```python
from build123d import *

# Parameters (mm, degrees)
BOSS_EXTRUDE1_DEPTH                        = 3
SKETCH4_R                                  = 2.250000000000006
CUT_EXTRUDE2_DEPTH                         = 3
MIRROR1_AT_THE_SECOND_PLANE_COPY_1_SKETC_R = 2.250000000000006
MIRROR1_AT_THE_SECOND_PLANE_COPY_1_DEPTH   = 3
FILLET4_R                                  = 1
CUT_EXTRUDE3_DEPTH                         = 1
SKETCH6_W                                  = 27.499999999999993
SKETCH6_H                                  = 27.999999999999996
CUT_EXTRUDE4_DEPTH                         = 1
CUT_EXTRUDE5_DEPTH                         = 3
SKETCH8_W                                  = 13.499999999999996
SKETCH8_H                                  = 13.700000000000003
CUT_EXTRUDE6_DEPTH                         = 1
SKETCH9_W                                  = 13.5
SKETCH9_H                                  = 3.5000000000000036
CUT_EXTRUDE7_DEPTH                         = 3
SKETCH10_W                                 = 13.499999999999996
SKETCH10_H                                 = 3.5000000000000036
SKETCH10_H_2                               = 3.5000000000000018
CUT_EXTRUDE8_DEPTH                         = 3
BOSS_EXTRUDE2_DEPTH                        = 23.5
CUT_EXTRUDE9_DEPTH                         = 29
SKETCH13_W                                 = 20.500000000000004
SKETCH13_H                                 = 6.0000000000000036
CUT_EXTRUDE10_DEPTH                        = 3
FILLET5_R                                  = 1
FILLET6_R                                  = 1
SKETCH14_W                                 = 20.8
SKETCH14_H                                 = 3.0000000000000036
CUT_EXTRUDE11_DEPTH                        = 1


with BuildPart() as part:
    # Sketch1 → Boss-Extrude1 (new body)
    with BuildSketch(Plane(origin=(0, 0, 0), x_dir=(1, 0, 0), z_dir=(0, 1, 0))):
        Polygon((-35, 35.00000000000001), (35, 35.00000000000001), (35.000000000000014, -34.99999999999999), (-35, -34.99999999999999), align=None)
    extrude(amount=BOSS_EXTRUDE1_DEPTH)

    # Sketch4 → Cut-Extrude2 (cut)
    with BuildSketch(Plane(origin=(0, 0, 0), x_dir=(-1, 0, 0), z_dir=(0, -1, 0))):
        with Locations(Location((30.500000000000004, -30.499999999999993, 0), (0, 0, 90))):
            Circle(SKETCH4_R)
    cut_extrude2 = extrude(amount=-CUT_EXTRUDE2_DEPTH, mode=Mode.SUBTRACT)

    # Mirror1: Cut-Extrude2 across plane
    add(cut_extrude2.mirror(Plane(origin=(0, 0, 0), x_dir=(0, 0, 1), z_dir=(1, 0, 0))), mode=Mode.SUBTRACT)

    # Mirror1 at the second plane: Cut-Extrude2 across plane
    add(cut_extrude2.mirror(Plane.XY), mode=Mode.SUBTRACT)

    # Mirror1 at the second plane copy 1 sketc → Mirror1 at the second plane copy 1 (cut)
    with BuildSketch(Plane.XZ):
        with Locations(Location((30.500000000000004, -30.499999999999993, 0), (0, 0, 90))):
            Circle(MIRROR1_AT_THE_SECOND_PLANE_COPY_1_SKETC_R)
    extrude(amount=-MIRROR1_AT_THE_SECOND_PLANE_COPY_1_DEPTH, mode=Mode.SUBTRACT)

    # Fillet4
    fillet4_edges = [part.edges().sort_by_distance(p)[0] for p in [
        (7.11e-15, 0, 34.99999999999999),
        (-35, 0, -7.11e-15),
        (0, 0, -35.00000000000001),
        (35.00000000000001, 0, -7.11e-15),
    ]]
    fillet(fillet4_edges, radius=FILLET4_R)

    # Sketch5 → Cut-Extrude3 (cut)
    with BuildSketch(Plane(origin=(0, 0, 0), x_dir=(-1, 0, 0), z_dir=(0, -1, 0))):
        Polygon((28.79465847473562, -24.725896818258043), (7.994658474735617, -24.725896818258047), (7.994658474735617, 20.774103181741953), (28.79465847473562, 20.774103181741957), align=None)
    extrude(amount=-CUT_EXTRUDE3_DEPTH, mode=Mode.SUBTRACT)

    # Sketch6 → Cut-Extrude4 (cut)
    with BuildSketch(Plane.XZ):
        with Locations((15.477858409688114, -6.209961428811168)):
            Rectangle(SKETCH6_W, SKETCH6_H)
    extrude(amount=-CUT_EXTRUDE4_DEPTH, mode=Mode.SUBTRACT)

    # Sketch7 → Cut-Extrude5 (cut)
    with BuildSketch(Plane(origin=(0, 1, 0), x_dir=(-1, 0, 0), z_dir=(0, -1, 0))):
        Polygon((-7.977858409688114, 15.209961428811162), (-22.977858409688114, 15.20996142881116), (-22.977858409688114, 20.209961428811166), (-7.977858409688114, 20.209961428811166), align=None)
    extrude(amount=-CUT_EXTRUDE5_DEPTH, mode=Mode.SUBTRACT)

    # Sketch8 → Cut-Extrude6 (cut)
    with BuildSketch(Plane.XZ):
        Polygon((-0.32931613637633694, 25.216207013959828), (13.170683863623664, 25.216207013959828), (13.170683863623664, 11.516207013959828), (-0.3293161363763353, 11.516207013959828), align=None)
        with Locations((23.356942305835496, 18.36620701395983)):
            Rectangle(SKETCH8_W, SKETCH8_H)
    extrude(amount=-CUT_EXTRUDE6_DEPTH, mode=Mode.SUBTRACT)

    # Sketch9 → Cut-Extrude7 (cut)
    with BuildSketch(Plane(origin=(0, 1, 0), x_dir=(-1, 0, 0), z_dir=(0, -1, 0))):
        with Locations((-6.420683863623664, -23.46620701395983)):
            Rectangle(SKETCH9_W, SKETCH9_H)
        Polygon((0.3293161363763353, -11.516207013959828), (-13.170683863623664, -11.51620701395983), (-13.170683863623664, -15.01620701395983), (0.3293161363763357, -15.016207013959828), align=None)
    extrude(amount=-CUT_EXTRUDE7_DEPTH, mode=Mode.SUBTRACT)

    # Sketch10 → Cut-Extrude8 (cut)
    with BuildSketch(Plane.XZ.offset(-1)):
        with Locations((23.356942305835496, 23.46620701395983)):
            Rectangle(SKETCH10_W, SKETCH10_H)
        with Locations((23.356942305835496, 13.266207013959828)):
            Rectangle(SKETCH10_W, SKETCH10_H_2)
    extrude(amount=-CUT_EXTRUDE8_DEPTH, mode=Mode.SUBTRACT)

    # Sketch11 → Boss-Extrude2 (add)
    with BuildSketch(Plane(origin=(0, 1, 0), x_dir=(-1, 0, 0), z_dir=(0, -1, 0))):
        Polygon((31.644658474735618, -26.345290910107266), (5.144658474735617, -26.34529091010727), (5.144658474735617, 5.654709089892729), (31.644658474735618, 5.654709089892732), align=None)
    extrude(amount=BOSS_EXTRUDE2_DEPTH)

    # Sketch12 → Cut-Extrude9 (cut)
    with BuildSketch(Plane(origin=(5.6e-16, 0, -5.654709089892728), x_dir=(-1, 0, -1e-16), z_dir=(1e-16, 0, -1))):
        Polygon((8.144658474735618, 1), (28.644658474735618, 1), (28.64465847473562, -19.5), (8.14465847473562, -19.5), align=None)
    extrude(amount=-CUT_EXTRUDE9_DEPTH, mode=Mode.SUBTRACT)

    # Sketch13 → Cut-Extrude10 (cut)
    with BuildSketch(Plane.XZ.offset(-1)):
        with Locations((-18.39465847473562, 20.345290910107273)):
            Rectangle(SKETCH13_W, SKETCH13_H)
    extrude(amount=-CUT_EXTRUDE10_DEPTH, mode=Mode.SUBTRACT)

    # Fillet5
    fillet5_edges = [part.edges().sort_by_distance(p)[0] for p in [
        (-5.144658474735617, -11.25, 26.34529091010727),
        (-31.644658474735618, -11.25, 26.345290910107266),
        (-5.144658474735617, -11.25, -5.654709089892729),
        (-31.644658474735618, -11.25, -5.654709089892732),
        (-28.64465847473562, -9.25, -5.654709089892731),
        (-18.39465847473562, -19.5, -5.65470908989273),
        (-8.144658474735618, -9.25, -5.654709089892729),
        (-18.394658474735618, -22.5, 26.345290910107266),
        (-5.144658474735617, -22.5, 10.34529091010727),
        (-18.394658474735618, -22.5, -5.65470908989273),
        (-31.644658474735618, -22.5, 10.345290910107268),
    ]]
    fillet(fillet5_edges, radius=FILLET5_R)

    # Fillet6
    fillet6_edges = [part.edges().sort_by_distance(p)[0] for p in [
        (-18.394658474735618, 0, 26.345290910107266),
        (-5.144658474735617, 0, 10.34529091010727),
        (-31.644658474735618, 0, 10.345290910107266),
        (-6.644658474735618, 0, -5.654709089892728),
        (-30.144658474735618, 0, -5.654709089892731),
        (-5.43755169354907, 0, 26.052397691293816),
        (-31.351765255922164, 0, 26.052397691293812),
        (-5.437551693549068, 0, -5.361815871079277),
        (-31.351765255922164, 0, -5.361815871079279),
        (-29.15823411660915, -8e-17, -5.528431782639838),
        (-7.631082832861968, 4e-17, -5.528431782639901),
    ]]
    fillet(fillet6_edges, radius=FILLET6_R)

    # Sketch14 → Cut-Extrude11 (cut)
    with BuildSketch(Plane.XZ):
        with Locations((-18.394658474735618, -22.274103181741957)):
            Rectangle(SKETCH14_W, SKETCH14_H)
    extrude(amount=-CUT_EXTRUDE11_DEPTH, mode=Mode.SUBTRACT)


solid = part.part
```
Read the model definition and answer for the solid it produces. Units are mm, in the model's axes. A direction names the side the tool comes from. Give positions to 0.01 mm unless a question says otherwise; leave off trailing zeros. Write each loop counter-clockwise with the first axis right and the second up, starting at its lowest first coordinate (ties: lowest second). Pieces come first, ordered by that corner, then holes. Notation, with made-up numbers: (51.25, 37) -> (82.25, 37) arc R26 ccw to (82.25, 64) -> close; hole circle Ø4 at (37.25, -13.75). An arc over 180 degrees is marked (long way). Answer in a Markdown table with one row per item.
1) A tool of negligible diameter and unlimited length cuts with its end or side. For faces 1 (the flat face through (30.107, 0.8, 18.3)), 2 (the flat face through (-19, -11, 26.345)), 3 (the flat face through (15, 2, -15.21)), 4 (the flat face through (-19, -19.5, 9)), from which of +Z, -Z, +X, -X, +Y, -Y can it reach the whole face along a straight path? Write none if from no direction.
Results list:
| item | result |
|---|---|
| face 1 | -Y |
| face 2 | +Z, +X, -X, -Y |
| face 3 | +Y, -Y |
| face 4 | -Z |
2) Section A-A on z = 30.5 is taken. Give the vertices of the cut face in (x, y).
Results list:
| item | result |
|---|---|
| outline | (-35, 1) arc R1 ccw to (-34, 0) -> (-32.75, 0) -> (-32.75, 3) -> (-35, 3) -> close; (-28.25, 0) -> (28.25, 0) -> (28.25, 3) -> (-28.25, 3) -> close; (32.75, 0) -> (34, 0) arc R1 ccw to (35, 1) -> (35, 3) -> (32.75, 3) -> close |
3) Determine the mould class of faces 5 (the flat face through (15, 1, -6)), 6 (the flat face through (-28.645, -8, 9)), 7 (the flat face through (35, 2, 0)) for opening direction Y: released by +Y, released by -Y, zero draft, split by the parting line, or undercut.
Results list:
| item | result |
|---|---|
| face 5 | released by -Y |
| face 6 | undercut |
| face 7 | zero draft |
4) Each of these flat-tipped pins is pushed along its axis until it touches: pin 1 Ø4 at (y, z) = (-14, -6.5) entering from -X; pin 2 Ø5 at (x, z) = (-30.5, 30.5) entering from -Y; pin 3 Ø7 at (y, z) = (-9.5, 8.5) entering from +X. Where does it stop, or does it pass through?
Results list:
| item | result |
|---|---|
| pin 1 | x = -31.64 |
| pin 2 | y = 0 |
| pin 3 | x = -5.14 |
5) Section D-D on z = 20.5 is taken. Give the vertices of the cut face in (x, y), plus the area to 3 significant figures.
Results list:
| item | result |
|---|---|
| outline | (-35, 1) arc R1 ccw to (-34, 0) -> (-32.64, 0) arc R1 cw to (-31.64, -1) -> (-31.64, -21.5) arc R1 ccw to (-30.64, -22.5) -> (-6.14, -22.5) arc R1 ccw to (-5.14, -21.5) -> (-5.14, -1) arc R1 cw to (-4.14, 0) -> (-0.33, 0) -> (-0.33, 1) -> (13.17, 1) -> (13.17, 0) -> (16.61, 0) -> (16.61, 1) -> (30.11, 1) -> (30.11, 0) -> (34, 0) arc R1 ccw to (35, 1) -> (35, 3) -> (-8.14, 3) -> (-8.14, -19.5) -> (-28.64, -19.5) -> (-28.64, 3) -> (-35, 3) -> close |
| area | 318 mm^2 |
6) Section B-B on x = 19 is taken. Give the vertices of the cut face in (y, z).
Results list:
| item | result |
|---|---|
| outline | (0, -34) arc R1 ccw to (1, -35) -> (3, -35) -> (3, -20.21) -> (0, -20.21) -> close; (0, 7.79) -> (1, 7.79) -> (1, -15.21) -> (3, -15.21) -> (3, 11.52) -> (0, 11.52) -> close; (0, 25.22) -> (3, 25.22) -> (3, 35) -> (1, 35) arc R1 ccw to (0, 34) -> close; (1, 15.02) -> (3, 15.02) -> (3, 21.72) -> (1, 21.72) -> close |
7) Section C-C on y = -7.75 is taken. Give the vertices of the cut face in (x, z), plus the area to 3 significant figures.
Results list:
| item | result |
|---|---|
| outline | (-31.64, -4.65) arc R1 ccw to (-30.64, -5.65) -> (-29.64, -5.65) arc R1 ccw to (-28.64, -4.65) -> (-28.64, 23.35) -> (-8.14, 23.35) -> (-8.14, -4.65) arc R1 ccw to (-7.14, -5.65) -> (-6.14, -5.65) arc R1 ccw to (-5.14, -4.65) -> (-5.14, 25.35) arc R1 ccw to (-6.14, 26.35) -> (-30.64, 26.35) arc R1 ccw to (-31.64, 25.35) -> close |
| area | 252 mm^2 |
8) Straight lines are drawn through the part: line 1 (X direction, y = 0.9, z = -30.5); line 2 (X direction, y = -9.25, z = 6.5); line 3 (Y direction, x = -9.5, z = 3.5). For each, find the intervals that lie inside material, in ascending order. Write a range as [from, to].
Results list:
| item | result |
|---|---|
| line 1 | [-34.99, -32.75], [-28.25, 28.25], [32.75, 34.99] |
| line 2 | [-31.64, -28.64], [-8.14, -5.14] |
| line 3 | [-22.5, -19.5], [1, 3] |
